from build123d import *

# Parameters (mm, degrees)
ESBO_O1_W                = 80
ESBO_O1_H                = 130
RESSALTO_EXTRUS_O1_DEPTH = 3
ESBO_O2_R                = 1.5
CORTE_EXTRUS_O1_DEPTH    = 3
ESBO_O2_3_R              = 1.5
CORTE_EXTRUS_O2_DEPTH    = 3
ESBO_O2_4_R              = 1.5
CORTE_EXTRUS_O3_DEPTH    = 3


with BuildPart() as part:
    # Esboço1 → Ressalto-extrusão1 (new body)
    with BuildSketch(Plane.XY):
        with Locations((-27.5, -29.311993606)):
            Rectangle(ESBO_O1_W, ESBO_O1_H)
    extrude(amount=RESSALTO_EXTRUS_O1_DEPTH)

    # Esboço2 → Corte-extrusão1 (cut)
    with BuildSketch(Plane.XY.offset(3)):
        with Locations((-55, 14.188006394)):
            Circle(ESBO_O2_R)
    extrude(amount=-CORTE_EXTRUS_O1_DEPTH, mode=Mode.SUBTRACT)

    # Esboço2<3> → Corte-extrusão2 (cut)
    with BuildSketch(Plane.XY.offset(3)):
        with Locations((0, 14.188006394)):
            Circle(ESBO_O2_3_R)
    extrude(amount=-CORTE_EXTRUS_O2_DEPTH, mode=Mode.SUBTRACT)

    # Esboço2<4> → Corte-extrusão3 (cut)
    with BuildSketch(Plane.XY.offset(3)):
        with Locations((0, -72.811993606)):
            Circle(ESBO_O2_4_R)
        with Locations((-55, -72.811993606)):
            Circle(ESBO_O2_4_R)
    extrude(amount=-CORTE_EXTRUS_O3_DEPTH, mode=Mode.SUBTRACT)


solid = part.part
Could you check a few things on this model? Use its own coordinates, in mm. Give positions to 0.01 mm unless a question says otherwise; leave off trailing zeros. Write each loop counter-clockwise with the first axis right and the second up, starting at its lowest first coordinate (ties: lowest second). Pieces come first, ordered by that corner, then holes. Notation, with made-up numbers: (-10.5, -28) -> (-4.5, -28) arc R7 ccw to (-4.5, -19) -> close; hole circle Ø1 at (66.25, 44). An arc over 180 degrees is marked (long way). Answer as CSV lines item,"result". Start each with the question number.
(1) I'm going to push a flat-ended pin straight in: pin 1 Ø2.5 at (x, y) = (0, 14.19) entering from -Z. Where does the tip first touch, or does it pass through?
(2) Please list where these lines run through material, in increasing order: line 1 (Y direction, x = -55, z = 1.65); line 2 (Y direction, x = -54.5, z = 2.4).
(3) If we mould it in two halves opening along Y, with no side actions, what happens to faces 1 (the face through (-28, -94.312, 1)), 2 (the face through (-54.308, -74.143, 1.521)), 3 (the face through (-67.5, -30, 1))? For each: +Y half, -Y half, draft (parallel to the pull), parting line (faces both ways), or undercut.
(4) If we section it at A-A, the plane x = -55: Write out the boundary of the cut face in (y, z), and give its area (3 significant figures).
Answer list:
1,pin 1,"through"
2,line 1,"-94.31 to -74.31, -71.31 to 12.69, 15.69 to 35.69"
2,line 2,"-94.31 to -74.23, -71.4 to 12.77, 15.6 to 35.69"
3,face 1,"-Y half"
3,face 2,"undercut"
3,face 3,"draft"
4,outline,"(-94.31, 0) -> (-74.31, 0) -> (-74.31, 3) -> (-94.31, 3) -> close; (-71.31, 0) -> (12.69, 0) -> (12.69, 3) -> (-71.31, 3) -> close; (15.69, 0) -> (35.69, 0) -> (35.69, 3) -> (15.69, 3) -> close"
4,area,"372 mm^2"
